For this review, use the dimensioned drawing (mm, ordinates from the lowest corner) and the shaded views. A direction names the side the tool comes from. Round coordinates to 2 decimals unless told otherwise and drop trailing zeros. Write each loop counter-clockwise with the first axis right and the second up, starting at its lowest first coordinate (ties: lowest second). Pieces come first, ordered by that corner, then holes.
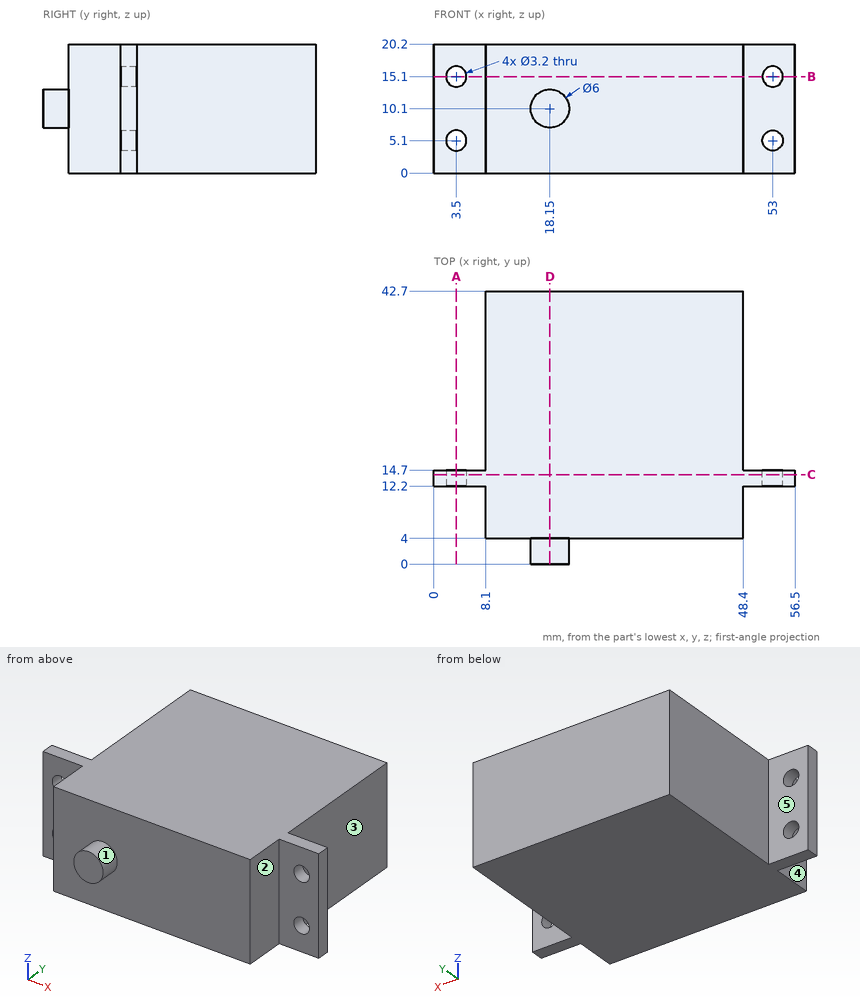
(1) For line 1 along X through (y, z) = (14.25, 5.1); line 2 along Z through (x, y) = (3.5, 13.6); line 3 along X through (y, z) = (5, 3), list the stretches that pass through material, from the lowest coordinate up.
Geometry check:
line 1: x = 0 to 1.9, 5.1 to 51.4, 54.6 to 56.5
line 2: z = 0 to 3.5, 6.7 to 13.5, 16.7 to 20.2
line 3: x = 8.1 to 48.4
(2) We need section D-D, the plane x = 18.15. Give the boundary of the cut face in (y, z).
Geometry check:
outline: (0, 7.1) - (4, 7.1) - (4, 0) - (42.7, 0) - (42.7, 20.2) - (4, 20.2) - (4, 13.1) - (0, 13.1) - close
(3) We need section A-A, the plane x = 3.5. Give the boundary of the cut face in (y, z).
Geometry check:
outline: (12.2, 0) - (14.7, 0) - (14.7, 3.5) - (12.2, 3.5) - close; (12.2, 6.7) - (14.7, 6.7) - (14.7, 13.5) - (12.2, 13.5) - close; (12.2, 16.7) - (14.7, 16.7) - (14.7, 20.2) - (12.2, 20.2) - close
(4) We need section C-C, the plane y = 14. Give the boundary of the cut face in (x, z), and give its area (3 significant figures).
Geometry check:
outline: (0, 0) - (56.5, 0) - (56.5, 20.2) - (0, 20.2) - close; hole circle Ø3.2 at (3.5, 5.1); hole circle Ø3.2 at (3.5, 15.1); hole circle Ø3.2 at (53, 5.1); hole circle Ø3.2 at (53, 15.1)
area: 1,110 mm2
(5) For the marked faces 1, 2, 3, 4 and 5, list the 3-axis set-ups (+Z, -Z, +X, -X, +Y, -Y) from which the entire face can be reached by the end or side of a thin tool; tool diameter is ignored.
Geometry check:
face 1: -Y
face 2: +Z, -Z, +X, -Y
face 3: +Z, -Z, +X, +Y
face 4: +Z, -Z, -X, -Y
face 5: +Z, -Z, -X, +Y
(6) We need section B-B, the plane z = 15.1. Give the boundary of the cut face in (x, y), and give its area (3 significant figures).
Geometry check:
outline: (0, 12.2) - (1.9, 12.2) - (1.9, 14.7) - (0, 14.7) - close; (5.1, 12.2) - (8.1, 12.2) - (8.1, 4) - (48.4, 4) - (48.4, 12.2) - (51.4, 12.2) - (51.4, 14.7) - (48.4, 14.7) - (48.4, 42.7) - (8.1, 42.7) - (8.1, 14.7) - (5.1, 14.7) - close; (54.6, 12.2) - (56.5, 12.2) - (56.5, 14.7) - (54.6, 14.7) - close
area: 1,580 mm2
(7) For pin 1 Ø12 at (x, z) = (15.5, 6.5) entering from -Y; pin 2 Ø2 at (y, z) = (31.5, 12) entering from +X; pin 3 Ø6.5 at (x, z) = (53, 10) entering from +Y; pin 4 Ø4 at (y, z) = (9, 14) entering from -X, all flat-tipped, find the tip position at first contact; note any pin that passes through.
Geometry check:
pin 1: stops at y = 0
pin 2: stops at x = 48.4
pin 3: stops at y = 14.7
pin 4: stops at x = 8.1
